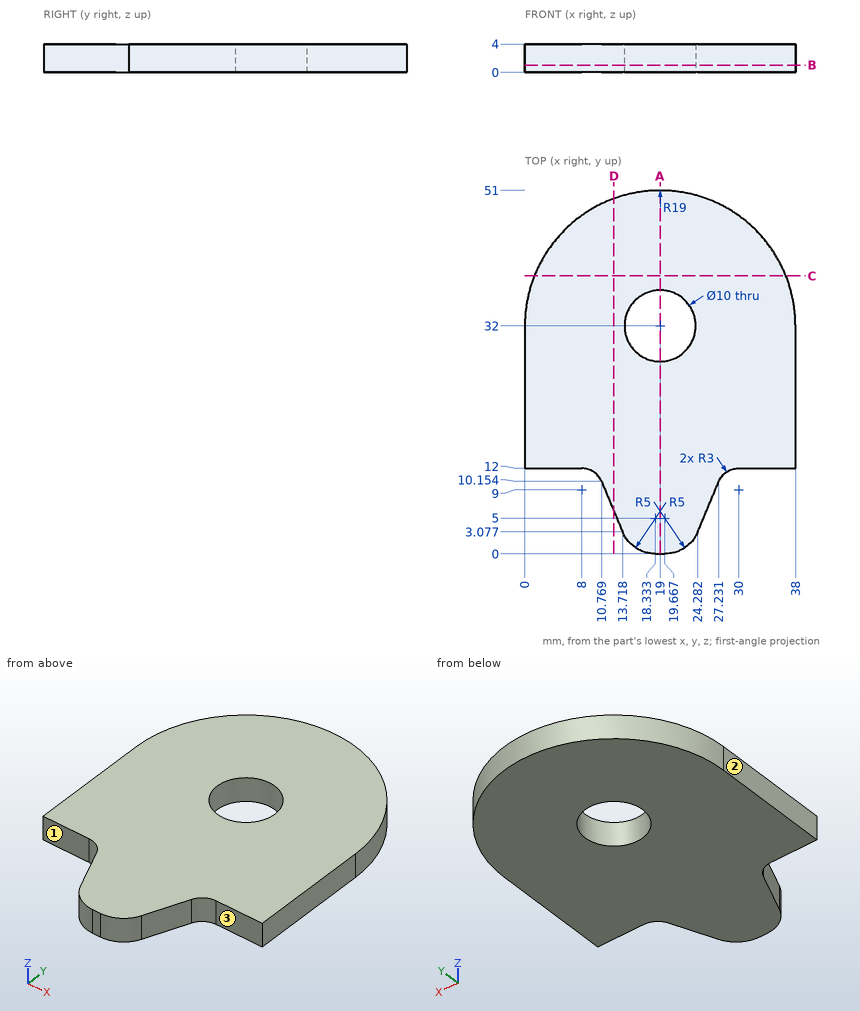
For this review, use the dimensioned drawing (mm, ordinates from the lowest corner) and the shaded views. A direction names the side the tool comes from. Round coordinates to 2 decimals unless told otherwise and drop trailing zeros. Order: outer loops, then holes, each group sorted by start corner. A loop starts at its lowest first (then second) coordinate and runs counter-clockwise, first axis right, second up. Notation, with made-up numbers: M 29,68.25 L 87,68.25 A31 ccw 87,104.25 Z; hole C -34,-19 d1. An arc over 180 degrees is marked long. Write each question's results on one line, items separated by ' | '. Start each with the question number.
1. Add section D-D (x = 12.5). State the section outline as (y, z) points.
2. Add section C-C (y = 39). State the section outline as (x, z) points, then the cut area to 3 significant figures.
3. Tool access review of the marked faces 1, 2 and 3: name each direction out of +Z, -Z, +X, -X, +Y, -Y from which nothing blocks a thin tool from reaching the whole face with its end or side.
4. To check wall thickness, follow L1, parallel to Y at x = 19, z = 1.15; L2, parallel to X at y = 33, z = 1.35; L3, parallel to X at y = 34, z = 0.9 (1 decimal). State the ranges of each line that lie inside material, in increasing order. Write a range as [from, to].
5. Add section B-B (z = 1.05). State the section outline as (x, y) points.
6. Add section A-A (x = 19). State the section outline as (y, z) points, then the cut area to 3 significant figures.
7. Clearance check with flat-ended pins moving along their axes: pin 1 Ø1.5 at (y, z) = (44, 3) entering from -X; pin 2 Ø2 at (x, z) = (33.5, 2) entering from +Y; pin 3 Ø2 at (x, z) = (21.5, 3) entering from +Y; pin 4 Ø16 at (x, y) = (19, 32) entering from -Z. State where each tip first meets the part, or that it passes through.
Output values:
1) outline: M 6,0 L 49.85,0 L 49.85,4 L 6,4 Z
2) outline: M 1.34,0 L 36.66,0 L 36.66,4 L 1.34,4 Z | area: 141 mm^2
3) face 1: +Z, -Z, -X, -Y | face 2: +Z, -Z, -X, +Y, -Y | face 3: +Z, -Z, +X, -Y
4) L1: [0, 27], [37, 51] | L2: [0.03, 14.1], [23.9, 37.97] | L3: [0.1, 14.4], [23.6, 37.9]
5) outline: M 0,12 L 8,12 A3 cw 10.77,10.15 L 13.72,3.08 A5 ccw 18.33,0 L 19.67,0 A5 ccw 24.28,3.08 L 27.23,10.15 A3 cw 30,12 L 38,12 L 38,32 A19 ccw 0,32 Z; hole C 19,32 d10
6) outline: M 0,0 L 27,0 L 27,4 L 0,4 Z; M 37,0 L 51,0 L 51,4 L 37,4 Z | area: 164 mm^2
7) pin 1: x = 3.69 | pin 2: y = 45.37 | pin 3: y = 50.94 | pin 4: z = 0
